from build123d import *

# Parameters (mm, degrees)
SKETCH_1_W                  = 47
SKETCH_1_H                  = 50
EXTRUDE_1_DEPTH             = 4
HOLE_WIZARD_3_5_3_5_1_D     = 3.5
HOLE_WIZARD_3_5_3_5_1_DEPTH = 4
FILLET_1_R                  = 2


with BuildPart() as part:
    # 草图1 → 凸台-拉伸1 (new body)
    with BuildSketch(Plane.XY):
        Rectangle(SKETCH_1_W, SKETCH_1_H)
    extrude(amount=EXTRUDE_1_DEPTH)

    # Ø3.5 (3.5) 直径孔1
    with Locations(Plane.XY.offset(4)):
        with Locations((-19, 21), (19, 21), (-19, -21), (19, -21)):
            Hole(HOLE_WIZARD_3_5_3_5_1_D / 2, depth=HOLE_WIZARD_3_5_3_5_1_DEPTH)

    # 圆角1
    fillet_1_edges = [part.edges().sort_by_distance(p)[0] for p in [
        (23.5, -25, 2),
        (-23.5, -25, 2),
        (-23.5, 25, 2),
        (23.5, 25, 2),
    ]]
    fillet(fillet_1_edges, radius=FILLET_1_R)


solid = part.part
Input: part model. Units: mm. Frame: model coordinates. Coordinates: 2 decimals unless noted, no trailing zeros. Order: outer loops, then holes, each group sorted by start corner. A loop starts at its lowest first (then second) coordinate and runs counter-clockwise, first axis right, second up. Notation, with made-up numbers: M -34.5,-33.5 L -5.5,-33.5 A9 ccw -5.5,-27.5 Z; hole C -26.75,-12 d9. An arc over 180 degrees is marked long. One line per question, with ' | ' between items.
Item 1: Section C-C (z = 2.1). Output: boundary loops of the cut face in (x, y).
Geometry results:
outline: M -23.5,-23 A2 ccw -21.5,-25 L 21.5,-25 A2 ccw 23.5,-23 L 23.5,23 A2 ccw 21.5,25 L -21.5,25 A2 ccw -23.5,23 Z; hole C -19,-21 d3.5; hole C -19,21 d3.5; hole C 19,-21 d3.5; hole C 19,21 d3.5
Item 2: Ray query, line 1 along Y through (x, z) = (19, 2.25); line 2 along X through (y, z) = (22, 1.35); line 3 along Y through (x, z) = (18, 1). Return the intervals inside material, ascending.
Geometry results:
line 1: y = -25 to -22.75, -19.25 to 19.25, 22.75 to 25 | line 2: x = -23.5 to -20.44, -17.56 to 17.56, 20.44 to 23.5 | line 3: y = -25 to -22.44, -19.56 to 19.56, 22.44 to 25
Item 3: Section A-A (x = 19). Output: boundary loops of the cut face in (y, z), then the cut area to 3 significant figures.
Geometry results:
outline: M -25,0 L -22.75,0 L -22.75,4 L -25,4 Z; M -19.25,0 L 19.25,0 L 19.25,4 L -19.25,4 Z; M 22.75,0 L 25,0 L 25,4 L 22.75,4 Z | area: 172 mm^2
Item 4: Draft query along X for faces 1 (the cylindrical face through (22.9, 24.43, 2.03)), 2 (the cylindrical face through (-18.772, 22.735, 1.972)), 3 (the cylindrical face through (-22.93, 24.4, 2.03)). Return one class per face: released by +X, released by -X, zero draft, split by the parting line, or undercut.
Geometry results:
face 1: released by +X | face 2: undercut | face 3: released by -X
Item 5: Section B-B (y = 21). Output: boundary loops of the cut face in (x, z).
Geometry results:
outline: M -23.5,0 L -20.75,0 L -20.75,4 L -23.5,4 Z; M -17.25,0 L 17.25,0 L 17.25,4 L -17.25,4 Z; M 20.75,0 L 23.5,0 L 23.5,4 L 20.75,4 Z
